Geometry check sheet. Reference: drawing and pictorial views, mm from the part's lowest x, y, z. A direction names the side the tool comes from. Give positions to 0.01 mm unless a question says otherwise; leave off trailing zeros. Order: outer loops, then holes, each group sorted by start corner. A loop starts at its lowest first (then second) coordinate and runs counter-clockwise, first axis right, second up. Notation, with made-up numbers: (39.25, 64.5) - (79.25, 64.5) arc R14 ccw to (79.25, 82.5) - close; hole circle Ø4 at (-26.5, 30). An arc over 180 degrees is marked (long way). Answer as a JSON object with one key per item and string values.
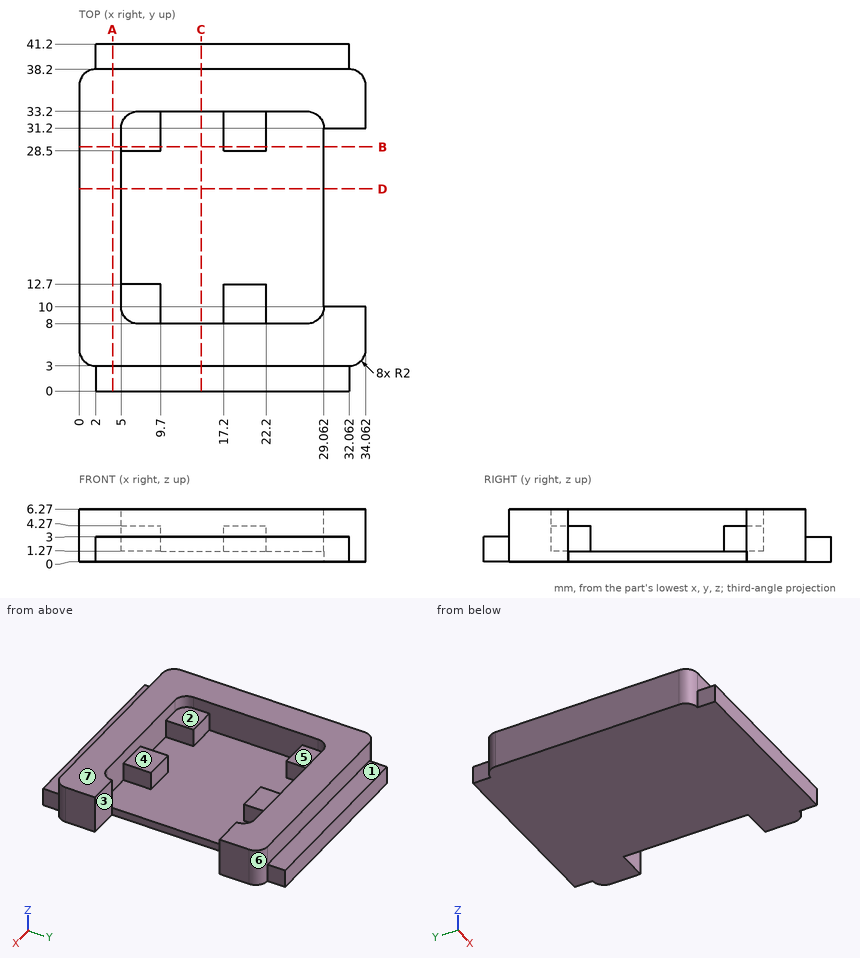
(1) Access from +Z, -Z, +X, -X, +Y, -Y to the whole of each face (thin tool, end or side, straight path). Record for the marked faces 1, 2 and 3.
Computed values:
{"face 1": "+Z, +X, -X, +Y", "face 2": "+Z", "face 3": "+Z, -Z, +X"}
(2) Section check A-A (x = 4). Record the cut outline in (y, z), then the cut area to 3 significant figures.
Computed values:
{"outline": "(0, 0) - (41.2, 0) - (41.2, 3) - (38.2, 3) - (38.2, 6.27) - (3, 6.27) - (3, 3) - (0, 3) - close", "area": "239 mm²"}
(3) Release check for a two-part mould opening along Y. For the marked faces 4, 5, 6 and 7 record: pulls with the +Y half, pulls with the -Y half, needs draft (parallel to the pull), parting line crosses it, or undercut.
Computed values:
{"face 4": "undercut", "face 5": "undercut", "face 6": "pulls with the +Y half", "face 7": "needs draft"}
(4) Gauge pin test, flat ends, axial feed: pin 1 Ø2.5 at (x, y) = (24.5, 39.5) entering from +Z; pin 2 Ø1.4 at (x, y) = (20, 10.5) entering from +Z; pin 3 Ø1.5 at (y, z) = (19.5, 2.5) entering from +X. Record the tip position at first contact, or that the pin passes through.
Computed values:
{"pin 1": "stops at z = 3", "pin 2": "stops at z = 4.27", "pin 3": "stops at x = 5"}
(5) Material ranges on line 1 along Y through (x, z) = (7, 5.25); line 2 along Y through (x, z) = (31, 3.75); line 3 along X through (y, z) = (12.5, 1.5), recorded low to high. Write a range as [from, to].
Computed values:
{"line 1": "y = [3, 8], [33.2, 38.2]", "line 2": "y = [3, 10], [31.2, 38.2]", "line 3": "x = [0, 9.7], [17.2, 22.2]"}
(6) Section check D-D (y = 24). Record the cut outline in (x, z).
Computed values:
{"outline": "(0, 0) - (29.06, 0) - (29.06, 1.27) - (5, 1.27) - (5, 6.27) - (0, 6.27) - close"}
(7) Section check C-C (x = 14.5). Record the cut outline in (y, z).
Computed values:
{"outline": "(0, 0) - (41.2, 0) - (41.2, 3) - (38.2, 3) - (38.2, 6.27) - (33.2, 6.27) - (33.2, 1.27) - (8, 1.27) - (8, 6.27) - (3, 6.27) - (3, 3) - (0, 3) - close"}
(8) Section check B-B (y = 29). Record the cut outline in (x, z).
Computed values:
{"outline": "(0, 0) - (29.06, 0) - (29.06, 1.27) - (22.2, 1.27) - (22.2, 4.27) - (17.2, 4.27) - (17.2, 1.27) - (9.7, 1.27) - (9.7, 4.27) - (5, 4.27) - (5, 6.27) - (0, 6.27) - close"}
